from build123d import *

# Parameters (mm, degrees)
F1_DEPTH = 63.5


with BuildPart() as f1:
    # F0 (on Front) → F1 (new body, symmetric)
    with BuildSketch(Plane.XZ):
        Polygon((-41.275, -9.525), (41.275, -9.525), (41.275, 9.525), (22.225, 9.525), (-41.275, 9.525), align=None)
        with BuildLine():
            Line((22.225, 9.525), (41.275, 9.525))
            Line((41.275, 9.525), (41.275, 34.049165))
            ThreePointArc((41.275, 34.049165), (43.860086, 40.290114), (50.101035, 42.8752))
            Line((50.101035, 42.8752), (55.933417, 42.8752))
            Line((55.933417, 42.8752), (55.933417, 61.9252))
            Line((55.933417, 61.9252), (50.101035, 61.9252))
            ThreePointArc((50.101035, 61.9252), (30.389702, 53.760498), (22.225, 34.049165))
            Line((22.225, 34.049165), (22.225, 9.525))
        make_face()
    extrude(amount=F1_DEPTH, both=True)


solid = f1.part
The listing builds one solid part. Answer for the finished solid, in the listing's coordinates (mm). A direction names the side the tool comes from. Give positions to 0.01 mm unless a question says otherwise; leave off trailing zeros. Write each loop counter-clockwise with the first axis right and the second up, starting at its lowest first coordinate (ties: lowest second). Pieces come first, ordered by that corner, then holes.
Item 1: Section A-A, the plane y = 9.5 is taken. Write down the section's boundary in (x, z) (3 decimals).
Item 2: Section B-B, the plane x = -10 is taken. Write down the section's boundary in (y, z) (3 decimals).
Item 3: Find the intervals of material crossed by line 1 along Z through (x, y) = (-31, 33) (3 decimals); line 2 along X through (y, z) = (-56, -6) (3 decimals); line 3 along X through (y, z) = (-39, 33.5) (3 decimals), in increasing order.
Item 4: Section C-C, the plane z = -5 is taken. Write down the section's boundary in (x, y) (3 decimals).
Item 5: Flat-ended cylindrical pins translate along their axes: P1, Ø2, axis at y = 27, z = 22.5, coming from the -X side (3 decimals); P2, Ø1.7, axis at x = 53.5, y = -24, coming from the -Z side; P3, Ø1.5, axis at x = -14, y = 26, coming from the +Z side (3 decimals). Find the tip coordinate at first contact, or state that the pin passes through.
Item 6: Which of the six approach directions +Z, -Z, +X, -X, +Y, -Y give full straight-line access (tool end or side, diameter ignored) to faces 1 (the flat face through (55.933, -1, 52)), 2 (the flat face through (53, -1, 42.875)), 3 (the flat face through (22.225, -1, 22))?
Completed:
1. outline: (-41.275, -9.525) - (41.275, -9.525) - (41.275, 34.049) arc R8.826 cw to (50.101, 42.875) - (55.933, 42.875) - (55.933, 61.925) - (50.101, 61.925) arc R27.876 ccw to (22.225, 34.049) - (22.225, 9.525) - (-41.275, 9.525) - close
2. outline: (-63.5, -9.525) - (63.5, -9.525) - (63.5, 9.525) - (-63.5, 9.525) - close
3. line 1: z = -9.525 to 9.525
3. line 2: x = -41.275 to 41.275
3. line 3: x = 22.225 to 41.275
4. outline: (-41.275, -63.5) - (41.275, -63.5) - (41.275, 63.5) - (-41.275, 63.5) - close
5. P1: stops at x = 22.225
5. P2: stops at z = 42.88
5. P3: stops at z = 9.525
6. face 1: +Z, -Z, +X, +Y, -Y
6. face 2: -Z, +X, +Y, -Y
6. face 3: +Z, -X, +Y, -Y
